Verification items for the finished model (mm, model axes). Coordinates: 2 decimals unless noted, no trailing zeros. Write each loop counter-clockwise with the first axis right and the second up, starting at its lowest first coordinate (ties: lowest second). Pieces come first, ordered by that corner, then holes. Notation, with made-up numbers: (38.5, 62.5) - (95.5, 62.5) arc R16 cw to (95.5, 66.5) - close; hole circle Ø8 at (34.25, 15). An arc over 180 degrees is marked (long way). Use one line per item in the form item = value. Start each with the question number.
(1) Material ranges on line 1 (Z direction, x = 16, y = -450); line 2 (Z direction, x = 16.5, y = -141), recorded low to high. Write a range as [from, to].
(2) Mould release check, pull along X, two halves, no side actions. Record for faces 1 (the flat face through (-19.05, -301, -5)), 2 (the cylindrical face through (2.842, -530.252, 27.142)), 3 (the flat face through (0, -609.6, 0)): released by +X, released by -X, zero draft, split by the parting line, or undercut.
(3) Sectioned sample at A-A (y = -422). Record the cut outline in (x, z), and give its area (3 significant figures).
(4) Gauge pin test, flat end, axial feed: pin 1 Ø6 at (x, y) = (-7.5, -359.5) entering from +Z. Record the tip position at first contact, or that the pin passes through.
from build123d import *

# Parameters (mm, degrees)
F1_DEPTH = 609.6
F3_R     = 3.175
F4_DEPTH = 25.4


with BuildPart() as f1:
    # F0 (on Front) → F1 (new body)
    with BuildSketch(Plane.XZ):
        Polygon((-19.05, -44.7250839726), (19.0490069268, -44.45), (19.0490069268, 44.45), (-19.05, 34.2392), align=None)
    extrude(amount=F1_DEPTH)

    # F3 (on face) → F4 (cut)
    with BuildSketch(Plane(origin=(-9.8380204896, 0, 36.7080748598), x_dir=(0.9659118691, 0, 0.2588711284), z_dir=(-0.2588711284, 0, 0.9659118691))):
        with Locations((10.1847013869, -76.2)):
            Circle(F3_R)
        with Locations((10.1847013869, -533.4)):
            Circle(F3_R)
    extrude(amount=-F4_DEPTH, mode=Mode.SUBTRACT)


solid = f1.part
Answers below:
q1.line_1 = [-44.47, 43.63]
q1.line_2 = [-44.47, 43.77]
q2.face_1 = released by -X
q2.face_2 = undercut
q2.face_3 = zero draft
q3.outline = (-19.05, -44.73) - (19.05, -44.45) - (19.05, 44.45) - (-19.05, 34.24) - close
q3.area = 3,200 mm2
q4.pin_1 = 38.14
